For this review, take the finished solid that the model builds, in its own axes (mm). Face numbers are marked on the shaded views. Coordinates: 2 decimals unless noted, no trailing zeros. Loops run counter-clockwise (first coordinate to the right, second up) from the corner with the lowest first, then second, coordinate; pieces in that order, holes last. Notation, with made-up numbers: M 6.25,27 L 17.25,27 A22 cw 17.25,61 Z; hole C 60,45.25 d8. An arc over 180 degrees is marked long. Answer as a JSON object with one key per item and string values. Group by question number.
Item 1: Add section D-D (y = -3.5). State the section outline as (x, z) points.
Item 2: Wall thickness on L1, parallel to Y at x = 0, z = -8.25; L2, parallel to Y at x = 0, z = -2; L3, parallel to Z at x = -0.25, y = -3: over which ranges is each line inside the solid? List them lowest first. Write a range as from..to.
Item 3: Insertion check: pin 1 (3 mm diameter, centred on x = -1, y = 0, fed in from -Z); pin 2 (1.5 mm diameter, centred on x = 2.5, z = 8.5, fed in from +Y); pin 3 (2 mm diameter, centred on y = 3.5, z = -1.5, fed in from +X). Each pin has a flat end and moves straight along its axis. Give the tip position at first contact, or say it passes through.
Item 4: Add section C-C (x = -1.75). State the section outline as (y, z) points.
Item 5: Add section B-B (y = 0). State the section outline as (x, z) points, then the cut area to 3 significant figures.
Item 6: Add section A-A (z = -2.75). State the section outline as (x, y) points, then the cut area to 3 significant figures.
Item 7: Mouldability with a two-part tool opening along Y and no side actions: class the marked faces 1, 2 and 3 as +Y half, -Y half, draft (parallel to the pull), parting line (faces both ways), or undercut.
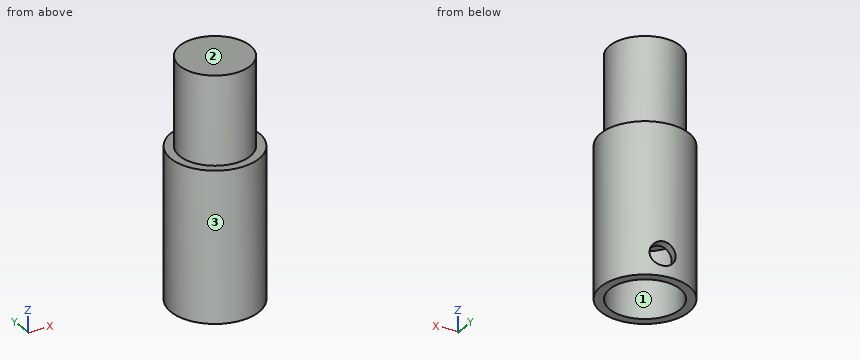
from build123d import *

# Parameters (mm, degrees)
BOSS_EXTRUDE1_DEPTH        = 13.5
BOSS_EXTRUDE1_DEPTH_BACK   = 13.5
SKETCH3_R                  = 5
SKETCH4_R                  = 5
SKETCH4_R_2                = 4
CUT_EXTRUDE1_DEPTH         = 10
CUT_EXTRUDE2_START         = -7.5
SKETCH5_R                  = 4
CUT_EXTRUDE2_DEPTH         = 7.5
SKETCH6_R                  = 3.1
CUT_EXTRUDE3_DEPTH         = 7
F_6_32_TAPPED_HOLE1_REACH  = 29.069
F_6_32_TAPPED_HOLE1_BORE_R = 1.35255


with BuildPart() as part:
    # Sketch3 → Boss-Extrude1 (new, two sides: drawn at the far end of the back side and taken through both)
    with BuildSketch(Plane.XY.offset(-BOSS_EXTRUDE1_DEPTH_BACK)):
        Circle(SKETCH3_R)
    extrude(amount=BOSS_EXTRUDE1_DEPTH + BOSS_EXTRUDE1_DEPTH_BACK)

    # Sketch4 → Cut-Extrude1 (cut)
    with BuildSketch(Plane.XY.offset(13.5)):
        Circle(SKETCH4_R)
        Circle(SKETCH4_R_2, mode=Mode.SUBTRACT)
    extrude(amount=-CUT_EXTRUDE1_DEPTH, mode=Mode.SUBTRACT)

    # Sketch5 → Cut-Extrude2 (cut)
    with BuildSketch(Plane(origin=(0, 0, -13.5), x_dir=(-1, 0, 0), z_dir=(0, 0, -1)).offset(CUT_EXTRUDE2_START)):
        with Locations(Location((0, 0, 0), (0, 0, 180))):
            Circle(SKETCH5_R)
    extrude(amount=CUT_EXTRUDE2_DEPTH, mode=Mode.SUBTRACT)

    # Sketch6 → Cut-Extrude3 (cut)
    with BuildSketch(Plane(origin=(0, 0, -6), x_dir=(-1, 0, 0), z_dir=(0, 0, -1))):
        Circle(SKETCH6_R)
    extrude(amount=-CUT_EXTRUDE3_DEPTH, mode=Mode.SUBTRACT)

    # #6-32 Tapped Hole1 bore (on position points) → #6-32 Tapped Hole1 (cut, up to next)
    with BuildSketch(Plane(origin=(0.817740869, 4.932676745, -11), x_dir=(0.986535349014, -0.163548173776, 0), z_dir=(0.163548173776, 0.986535349014, 0)), mode=Mode.PRIVATE) as f_6_32_tapped_hole1_sk1:
        Circle(F_6_32_TAPPED_HOLE1_BORE_R)
    f_6_32_tapped_hole1_tool1 = extrude(f_6_32_tapped_hole1_sk1.sketch, amount=-F_6_32_TAPPED_HOLE1_REACH, mode=Mode.PRIVATE) & part.part
    add(f_6_32_tapped_hole1_tool1.solids().sort_by_distance((0.817741, 4.932677, -11))[0], mode=Mode.SUBTRACT)


solid = part.part
From the geometry:
{
 "1": {"outline": "M -3.57,-13.5 L -1.94,-13.5 L -1.94,-6 L 1.94,-6 L 1.94,-13.5 L 3.57,-13.5 L 3.57,3.5 L 1.94,3.5 L 1.94,13.5 L -1.94,13.5 L -1.94,3.5 L -3.57,3.5 Z"},
 "2": {"L1": "y = -5..-4, 4..5", "L2": "y = -5..-3.1, 3.1..5", "L3": "z = 1..13.5"},
 "3": {"pin 1": "stops at z = 1", "pin 2": "stops at y = 3.6", "pin 3": "stops at x = 4.33"},
 "4": {"outline": "M -4.68,-13.5 L -3.6,-13.5 L -3.6,-6 L -2.56,-6 L -2.56,1 L 2.56,1 L 2.56,-6 L 3.6,-6 L 3.6,-13.5 L 4.68,-13.5 L 4.68,3.5 L 3.6,3.5 L 3.6,13.5 L -3.6,13.5 L -3.6,3.5 L -4.68,3.5 Z"},
 "5": {"outline": "M -5,-13.5 L -4,-13.5 L -4,-6 L -3.1,-6 L -3.1,1 L 3.1,1 L 3.1,-6 L 4,-6 L 4,-13.5 L 5,-13.5 L 5,3.5 L 4,3.5 L 4,13.5 L -4,13.5 L -4,3.5 L -5,3.5 Z", "area": "147 mm²"},
 "6": {"outline": "C 0,0 d10; hole C 0,0 d6.2", "area": "48.3 mm²"},
 "7": {"face 1": "undercut", "face 2": "draft", "face 3": "parting line"}
}
